Here's how the part is built. I have some questions about the finished solid (model axes, mm). A direction names the side the tool comes from. Coordinates: 2 decimals unless noted, no trailing zeros. Write each loop counter-clockwise with the first axis right and the second up, starting at its lowest first coordinate (ties: lowest second). Pieces come first, ordered by that corner, then holes.
from build123d import *

# Parameters (mm, degrees)
SKETCH1_W                                      = 6.5
SKETCH1_H                                      = 1
SKETCH1_R                                      = 1.75
SKETCH1_W_2                                    = 2
SKETCH1_H_2                                    = 12.5
SKETCH1_H_3                                    = 0.125
BOSS_EXTRUDE1_DEPTH                            = 2
SKETCH1_4_W                                    = 2
SKETCH1_4_H                                    = 12.5
BOSS_EXTRUDE2_DEPTH                            = 2.5
CSK_FOR_M2_FLAT_HEAD_MACHINE_SCREW2_AT_2_COUNT = 2
CSK_FOR_M2_FLAT_HEAD_MACHINE_SCREW2_AT_2_PITCH = 19.05
CSK_FOR_M2_FLAT_HEAD_MACHINE_SCREW2_AT_3_COUNT = 2
CSK_FOR_M2_FLAT_HEAD_MACHINE_SCREW2_AT_3_PITCH = 19.05
FILLET1_R                                      = 1


with BuildPart() as part:
    # Sketch1 → Boss-Extrude1 (new body)
    # profile 1 of 11: a face of its own
    with BuildSketch(Plane(origin=(0, 0, 0), x_dir=(1, 0, 0), z_dir=(0, 1, 0))):
        with Locations((0, 5.75)):
            Rectangle(SKETCH1_W, SKETCH1_H)
    # profile 2 of 11: a face of its own
    with BuildSketch(Plane(origin=(0, 0, 0), x_dir=(1, 0, 0), z_dir=(0, 1, 0))):
        Polygon((6.75, 6.25), (3.25, 6.25), (3.25, 5.25), (5.75, 5.25), (5.75, -5.25), (3.25, -5.25), (3.25, -6.25), (6.75, -6.25), align=None)
    # profile 3 of 11: a face of its own
    with BuildSketch(Plane(origin=(0, 0, 0), x_dir=(1, 0, 0), z_dir=(0, 1, 0))):
        Polygon((-3.25, 5.25), (-3.25, 6.25), (-6.75, 6.25), (-6.75, -6.25), (-3.25, -6.25), (-3.25, -5.25), (-5.75, -5.25), (-5.75, 5.25), align=None)
    # profile 4 of 11: a face of its own
    with BuildSketch(Plane(origin=(0, 0, 0), x_dir=(1, 0, 0), z_dir=(0, 1, 0))):
        with Locations((0, -5.75)):
            Rectangle(SKETCH1_W, SKETCH1_H)
    # profile 5 of 11: a face of its own
    with BuildSketch(Plane(origin=(0, 0, 0), x_dir=(1, 0, 0), z_dir=(0, 1, 0))):
        with BuildLine():
            Line((3.25, -9.525), (3.25, -6.375))
            Line((3.25, -6.375), (-3.25, -6.375))
            Line((-3.25, -6.375), (-3.25, -9.525))
            ThreePointArc((-3.25, -9.525), (0, -12.775), (3.25, -9.525))
        make_face()
        with Locations((0, -9.525)):
            Circle(SKETCH1_R, mode=Mode.SUBTRACT)
    # profile 6 of 11: a face of its own
    with BuildSketch(Plane(origin=(0, 0, 0), x_dir=(1, 0, 0), z_dir=(0, 1, 0))):
        with BuildLine():
            Line((3.25, 6.375), (3.25, 9.525))
            ThreePointArc((3.25, 9.525), (0, 12.775), (-3.25, 9.525))
            Line((-3.25, 9.525), (-3.25, 6.375))
            Line((-3.25, 6.375), (3.25, 6.375))
        make_face()
        with Locations((0, 9.525)):
            Circle(SKETCH1_R, mode=Mode.SUBTRACT)
    # profile 7 of 11: a face of its own
    with BuildSketch(Plane(origin=(0, 0, 0), x_dir=(1, 0, 0), z_dir=(0, 1, 0))):
        with Locations((-7.75, 0)):
            Rectangle(SKETCH1_W_2, SKETCH1_H_2)
    # profile 8 of 11: a face of its own
    with BuildSketch(Plane(origin=(0, 0, 0), x_dir=(1, 0, 0), z_dir=(0, 1, 0))):
        with Locations((0, 9.525)):
            Circle(SKETCH1_R)
    # profile 9 of 11: a face of its own
    with BuildSketch(Plane(origin=(0, 0, 0), x_dir=(1, 0, 0), z_dir=(0, 1, 0))):
        with Locations((0, -9.525)):
            Circle(SKETCH1_R)
    # profile 10 of 11: a face of its own
    with BuildSketch(Plane(origin=(0, 0, 0), x_dir=(1, 0, 0), z_dir=(0, 1, 0))):
        with Locations((0, -6.3125)):
            Rectangle(SKETCH1_W, SKETCH1_H_3)
    # profile 11 of 11: a face of its own
    with BuildSketch(Plane(origin=(0, 0, 0), x_dir=(1, 0, 0), z_dir=(0, 1, 0))):
        with Locations((0, 6.3125)):
            Rectangle(SKETCH1_W, SKETCH1_H_3)
    extrude(amount=BOSS_EXTRUDE1_DEPTH)

    # Sketch1_4 → Boss-Extrude2 (add)
    with BuildSketch(Plane(origin=(0, 0, 0), x_dir=(1, 0, 0), z_dir=(0, 1, 0))):
        with Locations((-7.75, 0)):
            Rectangle(SKETCH1_4_W, SKETCH1_4_H)
    extrude(amount=-BOSS_EXTRUDE2_DEPTH)

    # Sketch3 → CSK for M2 Flat Head Machine Screw2 (revolve, cut)
    with BuildSketch(Plane(origin=(0, 2, -9.525), x_dir=(0, 0, 1), z_dir=(1, 0, 0))):
        Polygon((0, 0), (0, 4.5), (1.2, 4.5), (1.2, 1), (2.2, 0), align=None)
    csk_for_m2_flat_head_machine_screw2 = revolve(axis=Axis((0, 8.35, -9.525), (0, -1, 0)), mode=Mode.SUBTRACT)

    # CSK for M2 Flat Head Machine Screw2 at 2: CSK for M2 Flat Head Machine Screw2 ×2
    with Locations(*[(0, 0, i * CSK_FOR_M2_FLAT_HEAD_MACHINE_SCREW2_AT_2_PITCH) for i in range(1, CSK_FOR_M2_FLAT_HEAD_MACHINE_SCREW2_AT_2_COUNT)]):
        add(csk_for_m2_flat_head_machine_screw2, mode=Mode.SUBTRACT)

    # CSK for M2 Flat Head Machine Screw2 at 3: CSK for M2 Flat Head Machine Screw2 ×2
    with Locations(*[(0, 0, i * CSK_FOR_M2_FLAT_HEAD_MACHINE_SCREW2_AT_3_PITCH) for i in range(1, CSK_FOR_M2_FLAT_HEAD_MACHINE_SCREW2_AT_3_COUNT)]):
        add(csk_for_m2_flat_head_machine_screw2, mode=Mode.SUBTRACT)

    # Fillet1
    fillet1_edges = [part.edges().sort_by_distance(p)[0] for p in [
        (5.75, 1, -5.25),
        (-5.75, 1, -5.25),
        (-5.75, 1, 5.25),
        (5.75, 1, 5.25),
        (-8.75, -0.25, 6.25),
        (-8.75, -0.25, -6.25),
        (-3.25, 1, -6.25),
        (3.25, 1, -6.25),
        (6.75, 1, -6.25),
        (6.75, 1, 6.25),
        (3.25, 1, 6.25),
        (-3.25, 1, 6.25),
    ]]
    fillet(fillet1_edges, radius=FILLET1_R)


solid = part.part
1. On a 3-axis mill with a long thin cutter (end or side, diameter ignored), from which of +Z, -Z, +X, -X, +Y, -Y can I reach the whole of each face in a straight line? I mean faces 4 (the face through (3.25, 1, 8)), 5 (the face through (3.25, 1, -8)), 6 (the face through (5.465, 1.014, -4.949)), 7 (the face through (-3.25, 1, 8)), 8 (the face through (-0.1, 0, 5.5)). Say none if no direction works.
2. I want a section at B-B (x = 0). List the corners of the cut face in (y, z) for me (3 decimals), then the cut area to 3 significant figures.
3. I want a section at C-C (x = -4.5). List the corners of the cut face in (y, z) for me.
4. I want a section at D-D (x = 5.25). List the corners of the cut face in (y, z) for me.
5. If I drill on line 1 (Z direction, x = 0, y = 0.6) (3 decimals); line 2 (X direction, y = 1.75, z = 3.75); line 3 (Y direction, x = 6, z = -5.25), over which ranges is the centre line in solid material (lowest first)?
6. I want a section at A-A (z = -3.5). List the corners of the cut face in (x, y) for me, then the cut area to 3 significant figures.
7. For pin 1 Ø1 at (x, y) = (-6.5, -1.5) entering from +Z; pin 2 Ø1 at (y, z) = (0.5, 8.5) entering from +X; pin 3 Ø1.6 at (x, y) = (5, 1) entering from +Z, each with a flat end and sliding along its axis, tell me the tip position at first contact or that it passes through.
8. Thinking about a two-plate mould opening in Z: for faces 1 (the face through (-3.551, 1.014, -6.535)), 2 (the face through (-5.449, 1.014, -4.965)), 3 (the face through (-8.75, 0, 0)), which applies, pulls with the +Z half, pulls with the -Z half, needs draft (parallel to the pull), parting line crosses it, or undercut?
Response values:
1. face 4: +Z, +X, +Y, -Y
1. face 5: -Z, +X, +Y, -Y
1. face 6: +Y, -Y
1. face 7: +Z, -X, +Y, -Y
1. face 8: +Z, -Z, +X, -Y
2. outline: (0, -12.775) - (2, -12.775) - (2, -11.725) - (1, -10.725) - (0, -10.725) - close; (0, -8.325) - (1, -8.325) - (2, -7.325) - (2, -5.25) - (0, -5.25) - close; (0, 5.25) - (2, 5.25) - (2, 7.325) - (1, 8.325) - (0, 8.325) - close; (0, 10.725) - (1, 10.725) - (2, 11.725) - (2, 12.775) - (0, 12.775) - close
2. area: 18.5 mm2
3. outline: (0, -6.25) - (2, -6.25) - (2, -5.25) - (0, -5.25) - close; (0, 5.25) - (2, 5.25) - (2, 6.25) - (0, 6.25) - close
4. outline: (0, -6.25) - (2, -6.25) - (2, -5.12) - (0, -5.12) - close; (0, 5.12) - (2, 5.12) - (2, 6.25) - (0, 6.25) - close
5. line 1: z = -12.775 to -10.725, -8.325 to -5.25, 5.25 to 8.325, 10.725 to 12.775
5. line 2: x = -8.75 to -5.75, 5.75 to 6.75
5. line 3: y = 0 to 2
6. outline: (-8.75, -2.5) - (-6.75, -2.5) - (-6.75, 0) - (-5.75, 0) - (-5.75, 2) - (-8.75, 2) - close; (5.75, 0) - (6.75, 0) - (6.75, 2) - (5.75, 2) - close
6. area: 13.0 mm2
7. pin 1: stops at z = 6.25
7. pin 2: stops at x = 3.25
7. pin 3: stops at z = 6.25
8. face 1: pulls with the -Z half
8. face 2: undercut
8. face 3: needs draft
